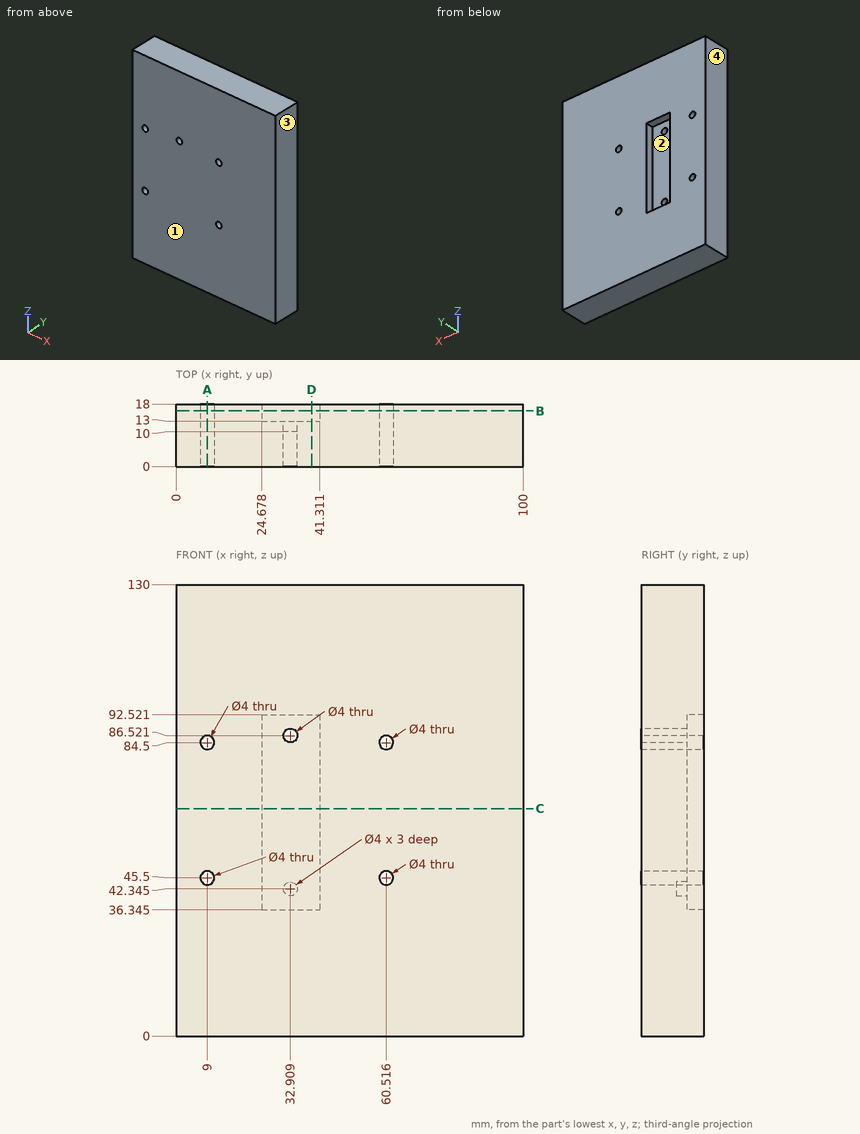
For this review, use the dimensioned drawing (mm, ordinates from the lowest corner) and the shaded views. Coordinates: 2 decimals unless noted, no trailing zeros. Order: outer loops, then holes, each group sorted by start corner. A loop starts at its lowest first (then second) coordinate and runs counter-clockwise, first axis right, second up. Notation, with made-up numbers: M 5,21 L 15,21 A11 cw 15,39 Z; hole C -23,-39 d3. An arc over 180 degrees is marked long. Answer as a JSON object with one key per item and string values. Group by question number.
1) Add section D-D, the plane x = 39. Write out the cut boundary in (y, z) (1 decimal), then the cut area to 3 significant figures.
2) For pin 1 (2.5 mm diameter, centred on x = 32.91, z = 42.34, fed in from +Y); pin 2 (2.5 mm diameter, centred on x = 60.52, z = 84.5, fed in from +Y); pin 3 (13.5 mm diameter, centred on x = 34.5, z = 62.5, fed in from +Y), all flat-tipped, find the tip position at first contact; note any pin that passes through.
3) Add section B-B, the plane y = 16. Write out the cut boundary in (x, z) (1 decimal), then the cut area to 3 significant figures.
4) Mouldability with a two-part tool opening along X and no side actions: class the marked faces 1, 2, 3 and 4 as pulls with the +X half, pulls with the -X half, needs draft (parallel to the pull), parting line crosses it, or undercut.
5) Wall thickness on L1, parallel to X at y = 14.5, z = 84.5; L2, parallel to X at y = 8, z = 45.5; L3, parallel to X at y = 14.5, z = 65.5: over which ranges is each line inside the solid? List them lowest first.
6) Add section C-C, the plane z = 65.5. Write out the cut boundary in (x, y), then the cut area to 3 significant figures.
7) Add section A-A, the plane x = 9. Write out the cut boundary in (y, z).
Computed values:
{
 "1": {"outline": "M 0,0 L 18,0 L 18,36.3 L 13,36.3 L 13,92.5 L 18,92.5 L 18,130 L 0,130 Z", "area": "2,060 mm^2"},
 "2": {"pin 1": "stops at y = 10", "pin 2": "passes through", "pin 3": "stops at y = 13"},
 "3": {"outline": "M 0,0 L 100,0 L 100,130 L 0,130 Z; hole C 9,45.5 d4; hole C 9,84.5 d4; hole M 24.7,36.3 L 41.3,36.3 L 41.3,92.5 L 24.7,92.5 Z; hole C 60.5,45.5 d4; hole C 60.5,84.5 d4", "area": "12,000 mm^2"},
 "4": {"face 1": "needs draft", "face 2": "undercut", "face 3": "pulls with the +X half", "face 4": "pulls with the -X half"},
 "5": {"L1": "x = 0 to 7, 11 to 24.68, 41.31 to 58.52, 62.52 to 100", "L2": "x = 0 to 7, 11 to 58.52, 62.52 to 100", "L3": "x = 0 to 24.68, 41.31 to 100"},
 "6": {"outline": "M 0,0 L 100,0 L 100,18 L 41.31,18 L 41.31,13 L 24.68,13 L 24.68,18 L 0,18 Z", "area": "1,720 mm^2"},
 "7": {"outline": "M 0,0 L 18,0 L 18,43.5 L 0,43.5 Z; M 0,47.5 L 18,47.5 L 18,82.5 L 0,82.5 Z; M 0,86.5 L 18,86.5 L 18,130 L 0,130 Z"}
}
